Verification items for the finished model (mm, model axes). Face numbers are marked on the shaded views. A direction names the side the tool comes from. Coordinates: 2 decimals unless noted, no trailing zeros. Order: outer loops, then holes, each group sorted by start corner. A loop starts at its lowest first (then second) coordinate and runs counter-clockwise, first axis right, second up.
Q1. Cross-section at C-C, the plane x = 93. Record the boundary of the cut face in (y, z).
Q2. Depth check by flat-ended pin: P1, Ø8, axis at x = 9.5, z = 69, coming from the -Y side; P2, Ø8.5, axis at y = 16.5, z = 34, coming from the -X side (3 decimals); P3, Ø3, axis at y = -49.5, z = 16.5, coming from the +X side (3 decimals). Enter the tip coordinate at first touch or a pass-through.
Q3. Cross-section at A-A, the plane z = 14. Record the boundary of the cut face in (x, y) (3 decimals).
Q4. Set-up check for the marked faces 1, 2, 3, 4 and 5: record each of +Z, -Z, +X, -X, +Y, -Y from which the full face is reachable in a straight line by a thin tool's end or side.
Q5. Cross-section at D-D, the plane y = -33. Record the boundary of the cut face in (x, z) (3 decimals), and give its area (3 significant figures).
Q6. Cross-section at B-B, the plane y = 12.5. Record the boundary of the cut face in (x, z) (3 decimals).
Q7. Thickness scan on line 1 (Y direction, x = -26, z = 40.5); line 2 (Y direction, x = 88, z = 80.5); line 3 (X direction, y = 18, z = 26) (3 decimals). Record the ranges inside material, lowest first.
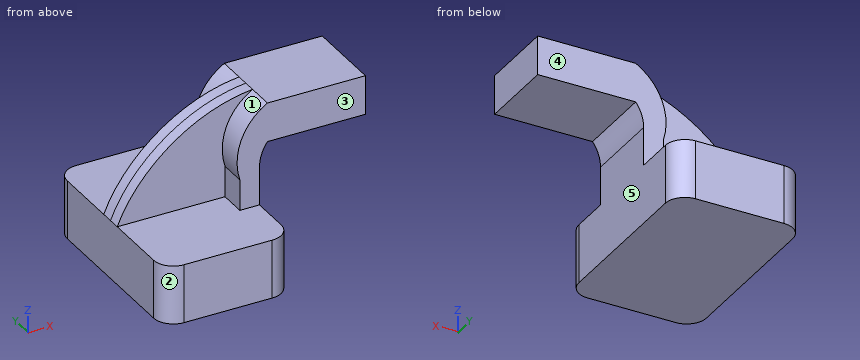
from build123d import *

# Parameters (mm, degrees)
F1_DEPTH = 63.5
F2_DEPTH = 25.4
F3_DEPTH = 7.9375
F4_R     = 12.7


with BuildPart() as f1:
    # F0 (on Front) → F1 (new body, symmetric)
    with BuildSketch(Plane.XZ):
        Polygon((-41.275, -19.05), (41.275, -19.05), (41.275, 19.05), (28.575, 19.05), (-41.275, 19.05), align=None)
    extrude(amount=F1_DEPTH, both=True)

    # F0 (on Front) → F2 (join, symmetric)
    with BuildSketch(Plane.XZ):
        with BuildLine():
            Line((28.575, 19.05), (41.275, 19.05))
            Line((41.275, 19.05), (41.275, 43.906411))
            ThreePointArc((41.275, 43.906411), (42.600833, 52.005452), (46.439918, 59.258983))
            Line((46.439918, 59.258983), (46.439918, 84.658983))
            ThreePointArc((46.439918, 84.658983), (29.442195, 65.035984), (28.575, 39.089256))
            Line((28.575, 39.089256), (28.575, 19.05))
        make_face()
        with BuildLine():
            Line((109.939918, 84.658983), (46.439918, 84.658983))
            Line((46.439918, 84.658983), (61.292269, 68.729509))
            ThreePointArc((61.292269, 68.729509), (53.018836, 65.322975), (46.439918, 59.258983))
            Line((46.439918, 59.258983), (109.939918, 59.258983))
            Line((109.939918, 59.258983), (109.939918, 84.658983))
        make_face()
        with BuildLine():
            Line((61.292269, 68.729509), (46.439918, 84.658983))
            Line((46.439918, 84.658983), (46.439918, 59.258983))
            ThreePointArc((46.439918, 59.258983), (53.018836, 65.322975), (61.292269, 68.729509))
        make_face()
    extrude(amount=F2_DEPTH, both=True)

    # F0 (on Front) → F3 (join, symmetric)
    with BuildSketch(Plane.XZ):
        with BuildLine():
            add(Edge.make_bspline(
                [(-41.275, 19.05), (-29.644612, 48.343893), (3.748323, 80.129104), (46.439918, 84.658983)],
                knots=[0, 0, 0, 0, 109.537416, 109.537416, 109.537416, 109.537416], degree=3))
            Line((-41.275, 19.05), (28.575, 19.05))
            Line((28.575, 19.05), (28.575, 39.089256))
            ThreePointArc((28.575, 39.089256), (29.442195, 65.035984), (46.439918, 84.658983))
        make_face()
    extrude(amount=F3_DEPTH, both=True)

    # F4
    f4_edges = [f1.edges().sort_by_distance(p)[0] for p in [
        (-41.275, -63.5, 0),
        (-41.275, 63.5, 0),
        (41.275, 63.5, 0),
        (41.275, -63.5, 0),
    ]]
    fillet(f4_edges, radius=F4_R)


solid = f1.part
Check values:
1. outline: (-25.4, 59.26) - (25.4, 59.26) - (25.4, 84.66) - (-25.4, 84.66) - close
2. P1: stops at y = -7.94
2. P2: stops at x = 28.575
2. P3: stops at x = 41.275
3. outline: (-41.275, -50.8) arc R12.7 ccw to (-28.575, -63.5) - (28.575, -63.5) arc R12.7 ccw to (41.275, -50.8) - (41.275, 50.8) arc R12.7 ccw to (28.575, 63.5) - (-28.575, 63.5) arc R12.7 ccw to (-41.275, 50.8) - close
4. face 1: -X, -Y
4. face 2: +Z, -Z, -X, -Y
4. face 3: +Z, +X, -X, -Y
4. face 4: +Z, +X, -X, +Y
4. face 5: -Z, +X, +Y, -Y
5. outline: (-41.275, -19.05) - (41.275, -19.05) - (41.275, 19.05) - (-41.275, 19.05) - close
5. area: 3,150 mm2
6. outline: (-41.275, -19.05) - (41.275, -19.05) - (41.275, 43.906) arc R25.4 cw to (46.44, 59.259) - (109.94, 59.259) - (109.94, 84.659) - (46.44, 84.659) arc R38.901 ccw to (28.575, 39.089) - (28.575, 19.05) - (-41.275, 19.05) - close
7. line 1: y = -7.94 to 7.94
7. line 2: y = -25.4 to 25.4
7. line 3: x = 28.575 to 41.275
